Geometry: final body of the model. Coordinates: model frame, mm. Face numbers are marked on the shaded views. A direction names the side the tool comes from. Give positions to 0.01 mm unless a question says otherwise; leave off trailing zeros. Loops run counter-clockwise (first coordinate to the right, second up) from the corner with the lowest first, then second, coordinate; pieces in that order, holes last.
1. Section B-B, the plane y = 10.5. Output: boundary loops of the cut face in (x, z).
2. Material intervals for line 1 along Y through (x, z) = (0, -3.25) (3 decimals); line 2 along Z through (x, y) = (-1, 6.5); line 3 along X through (y, z) = (8.5, 2), sorted ascending.
3. Access query for the marked faces 4, 5 and 6. Directions: +Z, -Z, +X, -X, +Y, -Y. A direction counts if a zero-diameter tool reaches every point of the face in a straight line with its end or side. Return the directions, or none.
4. First-contact query: P1, Ø1, axis at x = -1.5, y = 5.5, coming from the -Z side; P2, Ø4, axis at x = 5.5, z = 10.5, coming from the +Y side; P3, Ø5.5, axis at x = 0.5, z = -10, coming from the +Y side; P4, Ø2.5, axis at x = 0, y = 9.525, coming from the -Z side. Flat tips, straight axial feed; report the tip coordinate or a pass-through.
5. Section A-A, the plane x = 0. Output: boundary loops of the cut face in (y, z) (3 decimals), then the cut area to 3 significant figures.
6. Draft query along Y for the marked faces 1, 2 and 3. Return one class per face: +Y half, -Y half, draft (parallel to the pull), parting line (faces both ways), or undercut.
7. Section D-D, the plane z = -9.75. Output: boundary loops of the cut face in (x, y), then the cut area to 3 significant figures.
8. Section C-C, the plane z = -2.5. Output: boundary loops of the cut face in (x, y) (3 decimals).
from build123d import *

# Parameters (mm, degrees)
SKETCH1_W           = 25.4
SKETCH1_H           = 25.4
BOSS_EXTRUDE1_DEPTH = 2.54
SKETCH2_W           = 25.4
SKETCH2_H           = 12.7
BOSS_EXTRUDE2_DEPTH = 12.7
SKETCH3_R           = 1.5
CUT_EXTRUDE1_DEPTH  = 28.503637941
FILLET1_R           = 1.27


with BuildPart() as part:
    # Sketch1 → Boss-Extrude1 (new body)
    with BuildSketch(Plane(origin=(0, 0, 0), x_dir=(1, 0, 0), z_dir=(0, 1, 0))):
        Rectangle(SKETCH1_W, SKETCH1_H)
    extrude(amount=BOSS_EXTRUDE1_DEPTH)

    # Sketch2 → Boss-Extrude2 (add)
    with BuildSketch(Plane(origin=(0, 2.54, 0), x_dir=(1, 0, 0), z_dir=(0, 1, 0))):
        Rectangle(SKETCH2_W, SKETCH2_H)
    extrude(amount=BOSS_EXTRUDE2_DEPTH)

    # Sketch3 → Cut-Extrude1 (cut, through all)
    with BuildSketch(Plane.XY.offset(6.35)):
        with BuildLine():
            Line((-12.7, 2.54), (-2.102335281, 11.904245966))
            ThreePointArc((-2.102335281, 11.904245966), (0, 12.7), (2.102335281, 11.904245966))
            Line((2.102335281, 11.904245966), (12.7, 2.54))
            Line((12.7, 2.54), (12.7, 15.24))
            Line((12.7, 15.24), (-12.7, 15.24))
            Line((-12.7, 15.24), (-12.7, 2.54))
        make_face()
        with Locations((0, 9.525)):
            Circle(SKETCH3_R)
    extrude(amount=-CUT_EXTRUDE1_DEPTH, mode=Mode.SUBTRACT)

    # Fillet1
    fillet1_edges = [part.edges().sort_by_distance(p)[0] for p in [
        (0, 0, -12.7),
        (-12.7, 0, 0),
        (0, 0, 12.7),
        (12.7, 0, 0),
        (-12.7, 1.27, 12.7),
        (12.7, 1.27, 12.7),
        (-12.7, 1.27, -12.7),
        (12.7, 1.27, -12.7),
        (0, 2.54, -6.35),
        (0, 2.54, 6.35),
    ]]
    fillet(fillet1_edges, radius=FILLET1_R)


solid = part.part
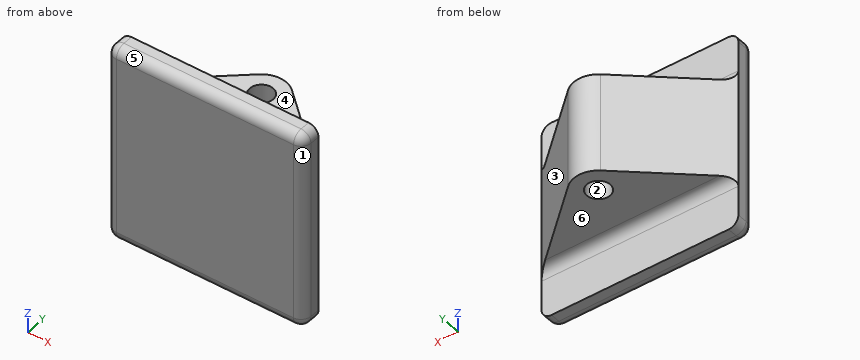
Answers below:
1. outline: (-3.69, -6.35) - (-1.14, -6.35) - (-1.14, 6.35) - (-3.69, 6.35) - close; (1.14, -6.35) - (3.69, -6.35) - (3.69, 6.35) - (1.14, 6.35) - close
2. line 1: y = 0 to 8.025, 11.025 to 12.7
2. line 2: z = -6.35 to 6.35
2. line 3: x = -5.95 to -1.1, 1.1 to 5.95
3. face 4: +Z, +X, -X, +Y
3. face 5: +Z, +X, -X, -Y
3. face 6: -Z, +X, -X, +Y
4. P1: stops at z = -6.35
4. P2: stops at y = 2.54
4. P3: stops at y = 2.6
4. P4: passes through
5. outline: (0, -11.43) arc R1.27 ccw to (1.27, -12.7) - (2.54, -12.7) - (2.54, -7.62) arc R1.27 cw to (3.81, -6.35) - (8.025, -6.35) - (8.025, 6.35) - (3.81, 6.35) arc R1.27 cw to (2.54, 7.62) - (2.54, 12.7) - (1.27, 12.7) arc R1.27 ccw to (0, 11.43) - close; (11.025, -6.35) - (12.7, -6.35) - (12.7, 6.35) - (11.025, 6.35) - close
5. area: 155 mm2
6. face 1: -Y half
6. face 2: undercut
6. face 3: +Y half
7. outline: (-12.7, 1.27) arc R1.27 ccw to (-11.43, 0) - (11.43, 0) arc R1.27 ccw to (12.7, 1.27) - (12.7, 2.54) - (-12.7, 2.54) - close
7. area: 63.8 mm2
8. outline: (-12.7, 1.27) arc R1.27 ccw to (-11.43, 0) - (11.43, 0) arc R1.27 ccw to (12.7, 1.27) - (12.7, 2.54) - (2.102, 11.904) arc R3.175 ccw to (-2.102, 11.904) - (-12.7, 2.54) - close; hole circle Ø3 at (0, 9.525)
